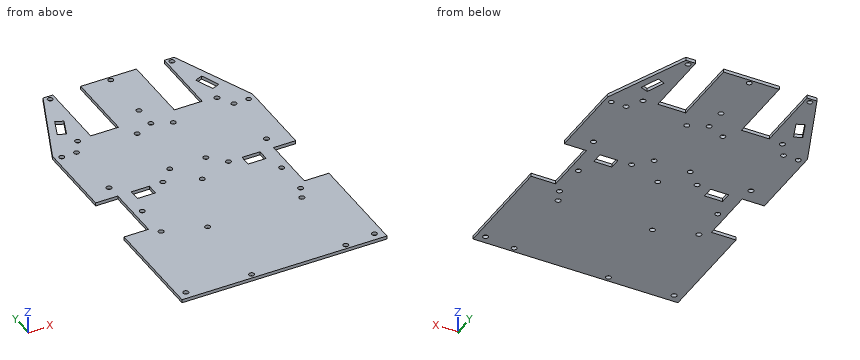
from build123d import *

# Parameters (mm, degrees)
SKETCH_1_R      = 1.6
SKETCH_1_W      = 11
SKETCH_1_H      = 7
SKETCH_1_R_2    = 1.5
EXTRUDE_1_DEPTH = 2


with BuildPart() as part:
    # 草圖1 → 填料-伸長1 (new body)
    with BuildSketch(Plane.XY):
        Polygon((62.5, 0), (62.5, 66), (47.5, 66), (47.5, 101), (61, 101), (61, 150), (40, 200), (34, 200), (34, 157), (17, 157), (17, 200), (-17, 200), (-17, 157), (-34, 157), (-34, 200), (-40, 200), (-61, 150), (-61, 101), (-47.5, 101), (-47.5, 66), (-62.5, 66), (-62.5, 0), align=None)
        with Locations((-18.5, 3)):
            Circle(SKETCH_1_R, mode=Mode.SUBTRACT)
        with Locations((-18.5, 53)):
            Circle(SKETCH_1_R, mode=Mode.SUBTRACT)
        with Locations((39, 3)):
            Circle(SKETCH_1_R, mode=Mode.SUBTRACT)
        with Locations((39, 53)):
            Circle(SKETCH_1_R, mode=Mode.SUBTRACT)
        Polygon((40.18903792, 175.844265317), (44.837242241, 177.686599868), (49.258845161, 166.530909498), (44.610640841, 164.688574948), align=None, mode=Mode.SUBTRACT)
        with Locations((0, 197.5)):
            Circle(SKETCH_1_R, mode=Mode.SUBTRACT)
        with Locations((37.09943713, 197.209058014)):
            Circle(SKETCH_1_R, mode=Mode.SUBTRACT)
        with Locations((-57.5, 5)):
            Circle(SKETCH_1_R, mode=Mode.SUBTRACT)
        with Locations((-42.5, 61)):
            Circle(SKETCH_1_R, mode=Mode.SUBTRACT)
        with Locations((-42.5, 82.5)):
            Circle(SKETCH_1_R, mode=Mode.SUBTRACT)
        with Locations((-33.75, 97.5)):
            Rectangle(SKETCH_1_W, SKETCH_1_H, mode=Mode.SUBTRACT)
        with Locations((57.5, 5)):
            Circle(SKETCH_1_R, mode=Mode.SUBTRACT)
        with Locations((42.5, 61)):
            Circle(SKETCH_1_R, mode=Mode.SUBTRACT)
        with Locations((0, 93.5)):
            Circle(SKETCH_1_R, mode=Mode.SUBTRACT)
        with Locations((42.5, 82.5)):
            Circle(SKETCH_1_R, mode=Mode.SUBTRACT)
        with Locations((33.75, 97.5)):
            Rectangle(SKETCH_1_W, SKETCH_1_H, mode=Mode.SUBTRACT)
        with Locations((-56.996650272, 147.008451352)):
            Circle(SKETCH_1_R, mode=Mode.SUBTRACT)
        with Locations((-20, 101)):
            Circle(SKETCH_1_R, mode=Mode.SUBTRACT)
        with Locations((-42.5, 156)):
            Circle(SKETCH_1_R, mode=Mode.SUBTRACT)
        Polygon((-44.837242241, 177.686599868), (-40.18903792, 175.844265317), (-44.610640841, 164.688574948), (-49.258845161, 166.530909498), align=None, mode=Mode.SUBTRACT)
        with Locations((-37.09943713, 197.209058014)):
            Circle(SKETCH_1_R, mode=Mode.SUBTRACT)
        with Locations((20, 101)):
            Circle(SKETCH_1_R, mode=Mode.SUBTRACT)
        with Locations((56.996650272, 147.008451352)):
            Circle(SKETCH_1_R_2, mode=Mode.SUBTRACT)
        with Locations((0, 152)):
            Circle(SKETCH_1_R, mode=Mode.SUBTRACT)
        with Locations((0, 165.5)):
            Circle(SKETCH_1_R, mode=Mode.SUBTRACT)
        with Locations((42.5, 156)):
            Circle(SKETCH_1_R, mode=Mode.SUBTRACT)
        with Locations((47.996650272, 110)):
            Circle(SKETCH_1_R, mode=Mode.SUBTRACT)
        with Locations((11, 147)):
            Circle(SKETCH_1_R, mode=Mode.SUBTRACT)
        with Locations((11, 110)):
            Circle(SKETCH_1_R, mode=Mode.SUBTRACT)
        with Locations((47.996650272, 147)):
            Circle(SKETCH_1_R, mode=Mode.SUBTRACT)
        with Locations((-11, 110)):
            Circle(SKETCH_1_R, mode=Mode.SUBTRACT)
        with Locations((-48, 147)):
            Circle(SKETCH_1_R, mode=Mode.SUBTRACT)
        with Locations((-48, 110)):
            Circle(SKETCH_1_R, mode=Mode.SUBTRACT)
        with Locations((-11, 147)):
            Circle(SKETCH_1_R, mode=Mode.SUBTRACT)
    extrude(amount=EXTRUDE_1_DEPTH)


solid = part.part
Work out the finished part from the listing and answer in its coordinate system (mm). Round coordinates to 2 decimals unless told otherwise and drop trailing zeros. Write each loop counter-clockwise with the first axis right and the second up, starting at its lowest first coordinate (ties: lowest second). Pieces come first, ordered by that corner, then holes.
1) Straight lines are drawn through the part: line 1 (Y direction, x = 11, z = 0.55); line 2 (Y direction, x = 0, z = 0.85); line 3 (X direction, y = 110, z = 0.5). For each, find the intervals that lie inside material, in ascending order.
2) A cutting plane is placed at C-C (x = -51.5). Give the vertices of the cut face in (y, z), plus the area to 3 significant figures.
3) A cutting plane is placed at D-D (z = 1.05). Give the number of separate pieces and of enclosed holes in the cut face, plus the area to 3 significant figures.
4) A cutting plane is placed at A-A (x = -32). Give the vertices of the cut face in (y, z), plus the area to 3 significant figures.
5) Given pin 1 Ø1 at (y, z) = (182.5, 1) entering from +X; pin 2 Ø0.6 at (x, z) = (54, 1.5) entering from +Y, each flat-ended and moving along its own axis, determine where each tip first touches the part or whether it passes through.
6) A cutting plane is placed at B-B (y = 137.5). Give the vertices of the cut face in (x, z), plus the area to 3 significant figures.
Completed:
1. line 1: y = 0 to 108.4, 111.6 to 145.4, 148.6 to 200
1. line 2: y = 0 to 91.9, 95.1 to 150.4, 153.6 to 163.9, 167.1 to 195.9, 199.1 to 200
1. line 3: x = -61 to -49.6, -46.4 to -12.6, -9.4 to 9.4, 12.6 to 46.4, 49.6 to 61
2. outline: (0, 0) - (66, 0) - (66, 2) - (0, 2) - close; (101, 0) - (172.62, 0) - (172.62, 2) - (101, 2) - close
2. area: 275 mm2
3. separate pieces: 1
3. enclosed holes: 34
3. area: 20,600 mm2
4. outline: (0, 0) - (94, 0) - (94, 2) - (0, 2) - close; (101, 0) - (157, 0) - (157, 2) - (101, 2) - close
4. area: 300 mm2
5. pin 1: stops at x = 47.56
5. pin 2: stops at y = 167.38
6. outline: (-61, 0) - (61, 0) - (61, 2) - (-61, 2) - close
6. area: 244 mm2
